Check sheet for the modelled part. Datum: model origin and axes. Units: mm. A direction names the side the tool comes from. Round coordinates to 2 decimals unless told otherwise and drop trailing zeros. Write each loop counter-clockwise with the first axis right and the second up, starting at its lowest first coordinate (ties: lowest second). Pieces come first, ordered by that corner, then holes.
Item 1: Section check C-C, the plane z = 176. Record the cut outline in (x, y), plus the area to 3 significant figures.
Item 2: Section check B-B, the plane x = 14. Record the cut outline in (y, z), plus the area to 3 significant figures.
Item 3: Release check for a two-part mould opening along Y. For faces 4 (the flat face through (-47, 76, 177)), 5 (the flat face through (-47, 80, 177)), 6 (the cylindrical face through (11.904, -48.458, 186.479)), 7 (the flat face through (-1, -48, 188)) record: pulls with the +Y half, pulls with the -Y half, needs draft (parallel to the pull), parting line crosses it, or undercut.
Item 4: Section check A-A, the plane y = 4. Record the cut outline in (x, z).
Item 5: Material ranges on line 1 along Y through (x, z) = (85, 185.95); line 2 along X through (y, z) = (-97, 186.6); line 3 along Z through (x, y) = (-67, 9.5), recorded low to high.
Item 6: Set-up check for faces 1 (the flat face through (-45, 78, 177)), 2 (the flat face through (-49, 78, 177)), 3 (the flat face through (-47, 78, 169)): record each of +Z, -Z, +X, -X, +Y, -Y from which the full face is reachable in a straight line by a thin tool's end or side.
Item 7: Depth check by flat-ended pin: pin 1 (3 mm diameter, centred on x = 85, y = 85, fed in from +Z); pin 2 (2 mm diameter, centred on x = -47, z = 175, fed in from -Y); pin 3 (2 mm diameter, centred on y = 79, z = 176, fed in from -X); pin 4 (4.5 mm diameter, centred on y = 79, z = 176.5, fed in from +X). Enter the tip coordinate at first touch or a pass-through.
Item 8: Section check D-D, the plane x = -41.5. Record the cut outline in (y, z).
from build123d import *

# Parameters (mm, degrees)
SKETCH244_R          = 1.85
PAD019_DEPTH         = 3
POCKET016_DEPTH      = 0.001
POCKET016_DEPTH_BACK = 3.001
SKETCH245_W          = 4
SKETCH245_H          = 16
PAD020_DEPTH         = 4


with BuildPart() as part:
    # Sketch244 → Pad019 (new body)
    with BuildSketch(Plane.XY):
        Polygon((91, 90), (-72, 90), (-72, -60), (-90, -60), (-90, -103), (91, -103), align=None)
        with Locations((85, 85)):
            Circle(SKETCH244_R, mode=Mode.SUBTRACT)
        with Locations((85, -97)):
            Circle(SKETCH244_R, mode=Mode.SUBTRACT)
        with Locations((-85, -97)):
            Circle(SKETCH244_R, mode=Mode.SUBTRACT)
    extrude(amount=PAD019_DEPTH)

    # Sketch243 → Pocket016 (cut, two sides)
    with BuildSketch(Plane.XY) as pocket016_sk:
        with BuildLine():
            ThreePointArc((-1, 54.311529), (14, -48.5), (29, 54.311529))
            Line((27.23673, 64.311529), (29, 54.311529))
            Line((0.76327, 64.311529), (27.23673, 64.311529))
            Line((-1, 54.311529), (0.76327, 64.311529))
        make_face()
    extrude(amount=-POCKET016_DEPTH, mode=Mode.SUBTRACT)
    extrude(pocket016_sk.sketch, amount=POCKET016_DEPTH_BACK, mode=Mode.SUBTRACT)

    # Sketch245 (on Face1 of Pocket016) → Pad020 (join)
    with BuildSketch(Plane(origin=(0, 80, 0), x_dir=(-1, 0, 0), z_dir=(0, 1, 0))):
        with Locations((47, -8)):
            Rectangle(SKETCH245_W, SKETCH245_H)
    extrude(amount=-PAD020_DEPTH)


with BuildPart() as part_1:
    # Body010 placement: moved
    add(part.part.moved(Location((0, 0, 185))))


solid = part_1.part
Values found:
1. outline: (-49, 76) - (-45, 76) - (-45, 80) - (-49, 80) - close
1. area: 16.0 mm2
2. outline: (-103, 185) - (-48.5, 185) - (-48.5, 188) - (-103, 188) - close; (64.31, 185) - (90, 185) - (90, 188) - (64.31, 188) - close
2. area: 241 mm2
3. face 4: pulls with the -Y half
3. face 5: pulls with the +Y half
3. face 6: undercut
3. face 7: needs draft
4. outline: (-72, 185) - (-38.5, 185) - (-38.5, 188) - (-72, 188) - close; (66.5, 185) - (91, 185) - (91, 188) - (66.5, 188) - close
5. line 1: y = -103 to -98.85, -95.15 to 83.15, 86.85 to 90
5. line 2: x = -90 to -86.85, -83.15 to 83.15, 86.85 to 91
5. line 3: z = 185 to 188
6. face 1: -Z, +X, +Y, -Y
6. face 2: -Z, -X, +Y, -Y
6. face 3: -Z, +X, -X, +Y, -Y
7. pin 1: passes through
7. pin 2: stops at y = 76
7. pin 3: stops at x = -49
7. pin 4: stops at x = -45
8. outline: (-103, 185) - (90, 185) - (90, 188) - (-103, 188) - close
